Input: part model. Units: mm. Frame: model coordinates. Face numbers are marked on the shaded views. Coordinates: 2 decimals unless noted, no trailing zeros. Loops run counter-clockwise (first coordinate to the right, second up) from the corner with the lowest first, then second, coordinate; pieces in that order, holes last. Notation, with made-up numbers: (5, 89.25) - (21, 89.25) arc R16 cw to (21, 104.25) - close; hole circle Ø5 at (31, 85). An arc over 180 degrees is marked (long way). Use a Markdown table: item, result. Add a question column.
1. Draft query along X for the marked faces 1, 2 and 3. Return one class per face: released by +X, released by -X, zero draft, split by the parting line, or undercut.
2. Contact query for flat-ended pins moving along their axis: P1, Ø1, axis at y = -13.5, z = 20.5, coming from the +X side; P2, Ø2, axis at y = -5, z = 33.5, coming from the -X side; P3, Ø10, axis at x = -18.5, y = -2, coming from the +Z side. Output: stop coordinate, or through.
3. Ray query, L1, parallel to Y at x = 0, z = 12; L2, parallel to X at y = 0, z = 9; L3, parallel to X at y = 4, z = 10.5. Return the intervals inside material, ascending. Write a range as [from, to].
4. Section query A-A on z = 37.5. Return the cut outline in (x, y).
```python
from build123d import *

# Parameters (mm, degrees)
F2_R     = 10.16
F3_R     = 10.16
F5_R     = 4.7752
F6_DEPTH = 10.795
F7_R     = 1.59385
F8_DEPTH = 20.32


# Not quite as in the source:
# - a fillet or chamfer that OpenCascade refuses, or shapes differently, is made with other operations: its cross-section is extruded or revolved along the edge and cut away or added


with BuildPart() as f1:
    # F0 (on Front) → F1 (revolve)
    with BuildSketch(Plane.XZ):
        Polygon((0, 50.8), (0, 0), (6.8085049027, 15.3191369531), (19.1836198036, 6.4245244719), (34.007973939, 27.0497159733), (10.633115835, 43.8503926785), (10.633115835, 50.8), align=None)
    revolve(axis=Axis((0, 0, 25.4), (0, 0, -1)))

    # F2
    f2_edges = [f1.edges().sort_by_distance(p)[0] for p in [
        (-10.633116, 0, 43.850393),
    ]]
    fillet(f2_edges, radius=F2_R)

    # F3
    f3_edges = [f1.edges().sort_by_distance(p)[0] for p in [
        (24.435674, 0, 33.929805),
        (-14.86337, 0, 40.809895),
        (-34.007974, 0, 27.049716),
    ]]
    fillet(f3_edges, radius=F3_R)

    # F4: fillet of radius 13.97 on 3 edges, made by hand

    # F4_s1 → F4_t2 (revolve, cut)
    with BuildSketch(Plane.XZ):
        with BuildLine():
            add(Edge.make_bspline(
                [(27.337014578, 17.7683797976), (19.1836198036, 6.4245244719), (7.8397644778, 14.5779192464)],
                knots=[0, 0, 0, 1, 1, 1], degree=2, weights=[1, 7.3333333333, 1]))
            Line((7.8397644778, 14.5779192464), (19.1836198036, 6.4245244719))
            Line((19.1836198036, 6.4245244719), (27.337014578, 17.7683797976))
        make_face()
    revolve(axis=Axis((0, 0, 6.4245244719), (0, 0, -1)), mode=Mode.SUBTRACT)

    # F5 (on face) → F6 (cut)
    with BuildSketch(Plane.XY.offset(50.8)):
        Circle(F5_R)
    extrude(amount=-F6_DEPTH, mode=Mode.SUBTRACT)

    # F7 (on Top) → F8 (cut)
    with BuildSketch(Plane.XY):
        Circle(F7_R)
    extrude(amount=F8_DEPTH, mode=Mode.SUBTRACT)


solid = f1.part
```
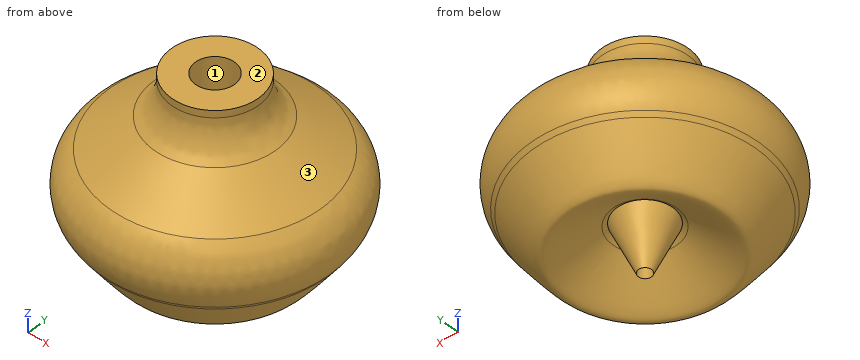
Resolved:
| question | item | result |
|---|---|---|
| 1 | face 1 | undercut |
| 1 | face 2 | zero draft |
| 1 | face 3 | split by the parting line |
| 2 | P1 | x = 26.1 |
| 2 | P2 | x = -25.91 |
| 2 | P3 | z = 41.88 |
| 3 | L1 | [-23.15, -11.44], [-5.33, -1.59], [1.59, 5.33], [11.44, 23.15] |
| 3 | L2 | [-20.82, -15.77], [-4, -1.59], [1.59, 4], [15.77, 20.82] |
| 3 | L3 | [-21.65, -12.97], [-2.4, 2.4], [12.97, 21.65] |
| 4 | outline | circle Ø38.94 at (0, 0) |
